Build history of the part. All positions in model axes, mm. A direction names the side the tool comes from. Round coordinates to 2 decimals unless told otherwise and drop trailing zeros. Write each loop counter-clockwise with the first axis right and the second up, starting at its lowest first coordinate (ties: lowest second). Pieces come first, ordered by that corner, then holes. Notation, with made-up numbers: M -20.5,51 L 5.5,51 A30 cw 5.5,89 Z; hole C 76.25,-6.75 d10. An arc over 180 degrees is marked long. Write item = value, one per line. Start each with the question number.
Q1. Band-saw the part on D-D on z = -102. Write the cut outline in (x, y).
Q2. Drop flat-ended pins along their axis: P1, Ø9.5, axis at x = 23.5, y = -3, coming from the +Z side; P2, Ø1.5, axis at x = 33, z = 7, coming from the -Y side; P3, Ø12, axis at x = 33, y = -8.5, coming from the -Z side. Give the stop position or say it passes through.
Q3. Pull direction X, two halves, no side cores. Call faces 1 (the cylindrical face through (23.642, -0.371, -122.977)), 2 (the cylindrical face through (20.24, 3.65, -9.24)), 3 (the flat face through (26, 26.5, -61)): released by +X, released by -X, zero draft, split by the parting line, or undercut.
Q4. Band-saw the part on A-A on y = 0. Write the cut outline in (x, z), plus the area to 3 significant figures.
Q5. Tool access for faces 4 (the flat face through (0, 0, -13)), 5 (the flat face through (25, 0, -44)), 6 (the flat face through (50, 0, -13)): list every direction of +Z, -Z, +X, -X, +Y, -Y with a clear straight run to the whole face (end or side of a thin tool).
Q6. Band-saw the part on C-C on x = 25. Write the cut outline in (y, z).
Q7. Band-saw the part on B-B on z = 15.5. Write the cut outline in (x, y), plus the area to 3 significant figures.
Q8. Probe L1, parallel to Y at x = 25, z = -11; L2, parallel to X at y = 0, z = -0.5; L3, parallel to X at y = 18.5, z = -23.5. List the from-to ranges inside material, lowest first.
Autodesk Inventor part; units mm, degrees
ref_plane "Work Plane1" through (25, 0, -44) normal (0, 0, 1) x (1, 0, 0)
ref_plane "YZ Plane" through (0, 0, 0) normal (1, 0, 0) x (0, 1, 0)
ref_plane "XZ Plane" through (0, 0, 0) normal (0, 1, 0) x (-1, 0, 0)
sketch "Sketch1" plane through (0, 0, 0) normal (0, 1, 0) x (-1, 0, 0)
  line L0 (0, 0) -> (-50, 0)
  line L1 (-50, 0) -> (-50, -83.5)
  line L2 (-50, -83.5) -> (0, -83.5)
  line L3 (0, -83.5) -> (0, 0)
  circle A0 centre (-25, -83.5) radius 39.5
  point P0 (-50, -52.9181)
  point P1 (0, -52.9181)
  dimension "d0" = 50
  dimension "d1" = 79
  dimension "d14" = 83.5
extrude "Extrusion1" add sketch "Sketch1" along normal mid plane 53
sketch "Sketch2" plane through (0, 0, 0) normal (1, 0, 0) x (0, 1, 0)
  line L0 (26.5, 0) -> (-26.5, 0)
  circle A0 centre (0, 0) radius 26.5
extrude "Extrusion2" add sketch "Sketch2" along normal up to surface (50 mm away) contours L0 A0 picked at (8.0782, 6.219)
ref_plane "Work Plane1" through (25, 0, -44) normal (0, 0, 1) x (1, 0, 0)
sketch "Sketch3" plane through (25, 0, -44) normal (0, 0, 1) x (1, 0, 0)
  circle A0 centre (0, 0) radius 6
  line L0 (-25, 0) -> (27.9863, 0) construction
  line L1 (39.5, 26.5) -> (-39.5, 26.5) construction
  line L2 (0, 26.5) -> (0, -26.5) construction
  point P0 (25, 26.5)
  point P1 (-25, 26.5)
  dimension "d15" = 12
extrude "Extrusion3" cut sketch "Sketch3" along normal through all
properties part number "thigh_inventor"
Conclusion:
q1.outline = M -9.9,-26.5 L 59.9,-26.5 L 59.9,26.5 L -9.9,26.5 Z
q2.P1 = 26.47
q2.P2 = -25.75
q2.P3 = -122.95
q3.face_1 = split by the parting line
q3.face_2 = undercut
q3.face_3 = zero draft
q4.outline = M 0,-52.92 A39.5 ccw long 50,-52.92 L 50,26.5 L 31,26.5 L 31,-44 L 19,-44 L 19,26.5 L 0,26.5 Z
q4.area = 7,720 mm^2
q5.face_4 = +Z, -X, +Y, -Y
q5.face_5 = +Z
q5.face_6 = +Z, +X, +Y, -Y
q6.outline = M -26.5,-123 L 26.5,-123 L 26.5,0 A26.5 ccw 6,25.81 L 6,-44 L -6,-44 L -6,25.81 A26.5 ccw -26.5,0 Z
q7.outline = M 0,-21.49 L 50,-21.49 L 50,21.49 L 0,21.49 Z; hole C 25,0 d12
q7.area = 2,040 mm^2
q8.L1 = -26.5 to -6, 6 to 26.5
q8.L2 = 0 to 19, 31 to 50
q8.L3 = 0 to 50
